Can you work these out from the model? Positions are in its coordinate system, mm. A direction names the side the tool comes from. Round coordinates to 2 decimals unless told otherwise and drop trailing zeros. Order: outer loops, then holes, each group sorted by start corner. A loop starts at its lowest first (then second) coordinate and runs counter-clockwise, first axis right, second up. Notation, with made-up numbers: M 40,73.5 L 91,73.5 A22 cw 91,108.5 Z; hole C -8.5,44.5 d6. An arc over 180 degrees is marked long. One line per question, with ' | ' between items.
```python
from build123d import *

# Parameters (mm, degrees)
EXTRUDE_1_DEPTH         = 12
SKETCH_2_R              = 1.5
CUT_EXTRUDE3_DEPTH      = 16
CUT_EXTRUDE3_DEPTH_BACK = 10


with BuildPart() as part:
    # 草图1 → 凸台-拉伸1 (new body)
    with BuildSketch(Plane.XY):
        Polygon((-11, 15), (11, 15), (11, 5), (23, 5), (23, 0), (6, 0), (6, 10), (-6, 10), (-6, 0), (-23, 0), (-23, 5), (-11, 5), align=None)
    extrude(amount=EXTRUDE_1_DEPTH)

    # 草图2 → Cut-Extrude3 (cut, two sides)
    with BuildSketch(Plane(origin=(0, 0, 0), x_dir=(1, 0, 0), z_dir=(0, 1, 0))) as cut_extrude3_sk:
        with Locations((-15, -6)):
            Circle(SKETCH_2_R)
        with Locations((15, -6)):
            Circle(SKETCH_2_R)
    extrude(amount=CUT_EXTRUDE3_DEPTH, mode=Mode.SUBTRACT)
    extrude(cut_extrude3_sk.sketch, amount=-CUT_EXTRUDE3_DEPTH_BACK, mode=Mode.SUBTRACT)


solid = part.part
```
(1) Thinking about a two-plate mould opening in X: for faces 4 (the flat face through (-17, 5, 6)), 5 (the flat face through (-11, 10, 6)), 6 (the cylindrical face through (-16.5, 2.46, 5.93)), which applies, released by +X, released by -X, zero draft, split by the parting line, or undercut?
Final values:
face 4: zero draft | face 5: released by -X | face 6: undercut
(2) Will these pins go through, and if not, where does the flat tip stop? pin 1 Ø6 at (x, z) = (2, 7) entering from -Y; pin 2 Ø2.5 at (x, z) = (-15, 6) entering from -Y; pin 3 Ø2 at (y, z) = (11, 4) entering from -X; pin 4 Ø6 at (x, z) = (-15.5, 3) entering from +Y.
Final values:
pin 1: y = 10 | pin 2: through | pin 3: x = -11 | pin 4: y = 5
(3) If we section it at C-C on z = 6: Please give me the cut outline in (x, y), plus the area to 3 significant figures.
Final values:
outline: M -23,0 L -16.5,0 L -16.5,5 L -23,5 Z; M -13.5,0 L -6,0 L -6,10 L 6,10 L 6,0 L 13.5,0 L 13.5,5 L 11,5 L 11,15 L -11,15 L -11,5 L -13.5,5 Z; M 16.5,0 L 23,0 L 23,5 L 16.5,5 Z | area: 300 mm^2
(4) Please list where these lines run through material, in increasing order: probe 1 along X at (y, z) = (1.2, 6); probe 2 along X at (y, z) = (2.75, 7.75); probe 3 along Z at (x, y) = (15, 2.1). Write a range as [from, to].
Final values:
probe 1: [-23, -16.5], [-13.5, -6], [6, 13.5], [16.5, 23] | probe 2: [-23, -6], [6, 23] | probe 3: [0, 4.5], [7.5, 12]
(5) If we section it at A-A on y = 1.5: Please give me the cut outline in (x, z).
Final values:
outline: M -23,0 L -6,0 L -6,12 L -23,12 Z; M 6,0 L 23,0 L 23,12 L 6,12 Z; hole C -15,6 d3; hole C 15,6 d3
(6) If we section it at B-B on x = -15: Please give me the cut outline in (y, z).
Final values:
outline: M 0,0 L 5,0 L 5,4.5 L 0,4.5 Z; M 0,7.5 L 5,7.5 L 5,12 L 0,12 Z
(7) On a 3-axis mill with a long thin cutter (end or side, diameter ignored), from which of +Z, -Z, +X, -X, +Y, -Y can I reach the whole of each face in a straight line? I mean faces 1 (the flat face through (17, 0, 6)), 2 (the flat face through (11, 10, 6)), 3 (the flat face through (0, 10, 6)). Say none if no direction works.
Final values:
face 1: +Z, -Z, +X, -X, -Y | face 2: +Z, -Z, +X, +Y | face 3: +Z, -Z, -Y
(8) If we section it at D-D on y = 6.75: Please give me the cut outline in (x, z).
Final values:
outline: M -11,0 L -6,0 L -6,12 L -11,12 Z; M 6,0 L 11,0 L 11,12 L 6,12 Z
